Build history of the part. All positions in model axes, mm. Face numbers are marked on the shaded views. A direction names the side the tool comes from. Round coordinates to 2 decimals unless told otherwise and drop trailing zeros. Use one line per item in the form item = value. Start each with the question number.
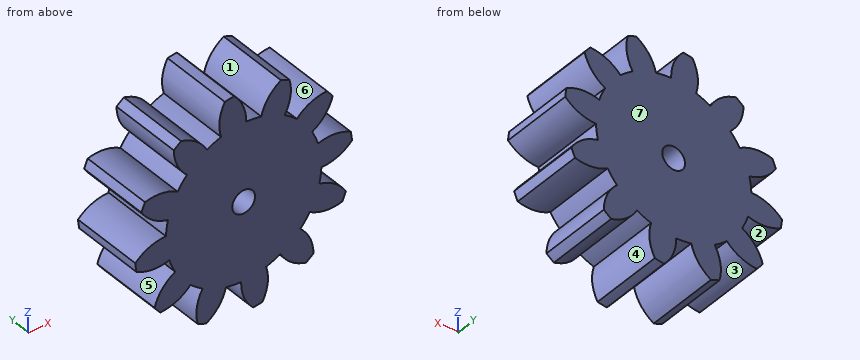
```python
from build123d import *

# Parameters (mm, degrees)
F2_DEPTH = 12.7
F3_COUNT = 12
F3_ANGLE = 330
F5_D     = 8


with BuildPart() as f2:
    # F1 (on Front) → F2 (new body, symmetric)
    with BuildSketch(Plane.XZ):
        with BuildLine():
            Line((0, 27.2142857143), (0, 32.6571428571))
            Line((0, 32.6571428571), (-4.1027982168, 31.163846429))
            Line((-4.1027982168, 31.163846429), (-3.5521770883, 26.9814637274))
            ThreePointArc((-3.5521770883, 26.9814637274), (-1.7798994455, 27.1560178396), (0, 27.2142857143))
        make_face()
        with BuildLine():
            Line((-3.5521770883, 26.9814637274), (-4.1027982168, 31.163846429))
            Line((-4.1027982168, 31.163846429), (-8.4908538679, 29.5667247857))
            ThreePointArc((-8.4908538679, 29.5667247857), (-8.2952422965, 27.7884140488), (-7.8836733992, 26.0473614916))
            ThreePointArc((-7.8836733992, 26.0473614916), (-5.7369683492, 26.6027167992), (-3.5521770883, 26.9814637274))
        make_face()
        with BuildLine():
            Line((-4.1027982168, 31.163846429), (-4.2626125059, 32.3777564729))
            ThreePointArc((-4.2626125059, 32.3777564729), (-6.3710925161, 32.0296450143), (-8.4522905301, 31.5443776985))
            ThreePointArc((-8.4522905301, 31.5443776985), (-8.5050911091, 30.5562048457), (-8.4908538679, 29.5667247857))
            Line((-8.4908538679, 29.5667247857), (-4.1027982168, 31.163846429))
        make_face()
        with BuildLine():
            ThreePointArc((-8.4522905301, 31.5443776985), (-6.3710925161, 32.0296450143), (-4.2626125059, 32.3777564729))
            Line((-4.2626125059, 32.3777564729), (-4.2993944212, 32.6571428571))
            Line((-4.2993944212, 32.6571428571), (-8.3117038653, 32.6571428571))
            ThreePointArc((-8.3117038653, 32.6571428571), (-8.3926831774, 32.1021103437), (-8.4522905301, 31.5443776985))
        make_face()
        with BuildLine():
            Line((-4.1027982168, 31.163846429), (0, 32.6571428571))
            ThreePointArc((0, 32.6571428571), (-2.1358793346, 32.5872214075), (-4.2626125059, 32.3777564729))
            Line((-4.2626125059, 32.3777564729), (-4.1027982168, 31.163846429))
        make_face()
        with BuildLine():
            ThreePointArc((-4.2626125059, 32.3777564729), (-2.1358793346, 32.5872214075), (0, 32.6571428571))
            Line((0, 32.6571428571), (-4.2993944212, 32.6571428571))
            Line((-4.2993944212, 32.6571428571), (-4.2626125059, 32.3777564729))
        make_face()
        with BuildLine():
            ThreePointArc((0, 32.6571428571), (-1.3922286837, 35.486786515), (-3.3594239194, 37.9516043262))
            ThreePointArc((-3.3594239194, 37.9516043262), (-4.1671816864, 37.8714219009), (-4.9730479236, 37.7740492183))
            Line((-4.9730479236, 37.7740492183), (-4.2993944212, 32.6571428571))
            Line((-4.2993944212, 32.6571428571), (0, 32.6571428571))
        make_face()
        with BuildLine():
            Line((-4.2993944212, 32.6571428571), (-4.9730479236, 37.7740492183))
            ThreePointArc((-4.9730479236, 37.7740492183), (-5.7766568393, 37.6595304772), (-6.5776436666, 37.5279176587))
            ThreePointArc((-6.5776436666, 37.5279176587), (-7.661923736, 35.1698741183), (-8.3117038653, 32.6571428571))
            Line((-8.3117038653, 32.6571428571), (-4.2993944212, 32.6571428571))
        make_face()
        with BuildLine():
            ThreePointArc((0.8734905136, 27.2002639925), (0.6971989167, 29.9703946199), (0, 32.6571428571))
            Line((0, 32.6571428571), (0, 27.2142857143))
            ThreePointArc((0, 27.2142857143), (0.4368015242, 27.210780058), (0.8734905136, 27.2002639925))
        make_face()
        with BuildLine():
            ThreePointArc((27.2142857143, 0), (23.1138516304, 14.3654867564), (12.0481915595, 24.4020168651))
            ThreePointArc((12.0481915595, 24.4020168651), (6.8095488061, 19.7367686343), (0, 18.0521428571))
            Line((0, 18.0521428571), (0, 0))
            Line((0, 0), (-2.402809942, 18.2511534992))
            ThreePointArc((-2.402809942, 18.2511534992), (-7.8527791982, 20.3429281496), (-12.0481915595, 24.4020168651))
            ThreePointArc((-12.0481915595, 24.4020168651), (-14.3654867564, -23.1138516304), (27.2142857143, 0))
        make_face()
        with BuildLine():
            ThreePointArc((-7.8836733992, 26.0473614916), (-9.9998299945, 25.3104868981), (-12.0481915595, 24.4020168651))
            ThreePointArc((-12.0481915595, 24.4020168651), (-7.8527791982, 20.3429281496), (-2.402809942, 18.2511534992))
            Line((-2.402809942, 18.2511534992), (-3.5521770883, 26.9814637274))
            ThreePointArc((-3.5521770883, 26.9814637274), (-5.7369683492, 26.6027167992), (-7.8836733992, 26.0473614916))
        make_face()
        with BuildLine():
            Line((0, 18.0521428571), (0, 27.2142857143))
            ThreePointArc((0, 27.2142857143), (-1.7798994455, 27.1560178396), (-3.5521770883, 26.9814637274))
            Line((-3.5521770883, 26.9814637274), (-2.402809942, 18.2511534992))
            ThreePointArc((-2.402809942, 18.2511534992), (-1.2055186491, 18.10198055), (0, 18.0521428571))
        make_face()
        with BuildLine():
            Line((0, 0), (0, 18.0521428571))
            ThreePointArc((0, 18.0521428571), (-1.2055186491, 18.10198055), (-2.402809942, 18.2511534992))
            Line((-2.402809942, 18.2511534992), (0, 0))
        make_face()
        with BuildLine():
            ThreePointArc((0.8734905136, 27.2002639925), (0.4368015242, 27.210780058), (0, 27.2142857143))
            Line((0, 27.2142857143), (0, 18.0521428571))
            ThreePointArc((0, 18.0521428571), (6.8095488061, 19.7367686343), (12.0481915595, 24.4020168651))
            ThreePointArc((12.0481915595, 24.4020168651), (6.6105985846, 26.399191906), (0.8734905136, 27.2002639925))
        make_face()
    extrude(amount=F2_DEPTH, both=True)

    # F3: F2 ×12 about axis
    f3_axis = Axis((0, 0, 0), (0, -1, 0))


with BuildPart() as f2_1:
    add(f2.part)
    for i in range(1, F3_COUNT):
        add(f2.part.rotate(f3_axis, i * F3_ANGLE / (F3_COUNT - 1)))

    # F5 (through all)
    with Locations(Plane.XZ.offset(12.7)):
        with Locations((0, 0)):
            Hole(F5_D / 2)


solid = f2_1.part
```
Q1. Drop flat-ended pins along their axis: P1, Ø3, axis at y = -5, z = 26.5, coming from the -X side; P2, Ø10, axis at y = 2.5, z = 27, coming from the -X side; P3, Ø4, axis at x = 25, y = -1.5, coming from the +Z side. Give the stop position or say it passes through.
Q2. Tool access for the marked faces 1, 2 and 3: list every direction of +Z, -Z, +X, -X, +Y, -Y with a clear straight run to the whole face (end or side of a thin tool).
Q3. Wall check: probe 1 along Z at (x, y) = (30, -0.5); probe 2 along Z at (x, y) = (-29.5, -9.25); probe 3 along Z at (x, y) = (-32, 2.75). Give the ranges that are in metal, low to high.
Q4. Pull direction Z, two halves, no side cores. Call the marked faces 4, 5, 6 and 7: pulls with the +Z half, pulls with the -Z half, needs draft (parallel to the pull), parting line crosses it, or undercut.
Filled in:
q1.P1 = -24.41
q1.P2 = -24.46
q1.P3 = 24.28
q2.face_1 = +Z, +Y, -Y
q2.face_2 = +Y, -Y
q2.face_3 = -Z, +Y, -Y
q3.probe_1 = -16.53 to -7.51, -0.69 to 8.51, 18.88 to 23.49
q3.probe_2 = -24.11 to -18.01, -8.49 to 0.76, 7.26 to 16.49
q3.probe_3 = -8.41 to 0.22, 8.78 to 16.5
q4.face_4 = undercut
q4.face_5 = undercut
q4.face_6 = pulls with the +Z half
q4.face_7 = needs draft
